Read the model definition and answer for the solid it produces. Units are mm, in the model's axes. A direction names the side the tool comes from. Give positions to 0.01 mm unless a question says otherwise; leave off trailing zeros. Loops run counter-clockwise (first coordinate to the right, second up) from the corner with the lowest first, then second, coordinate; pieces in that order, holes last. Notation, with made-up numbers: (21.25, 66) -> (39.25, 66) arc R13 cw to (39.25, 74) -> close; hole circle Ø7 at (57.25, 50.25). An arc over 180 degrees is marked (long way). Write each question's results on one line, items separated by ' | '. Start each with the question number.
Item 1: Find the intervals of material crossed by line 1 (Z direction, x = 6.5, y = 6); line 2 (Z direction, x = 51, y = 3.5); line 3 (Z direction, x = -26, y = 2.75), in increasing order.
Item 2: Which of the six approach directions +Z, -Z, +X, -X, +Y, -Y give full straight-line access (tool end or side, diameter ignored) to faces 1 (the flat face through (35, 3, 36.341)), 2 (the flat face through (-38.148, 3, 41))?
Item 3: Section B-B on y = 2.25 is taken. Write down the section's boundary in (x, z) (1 decimal).
Item 4: Each of these flat-tipped pins is pushed along its axis until it touches: P1, Ø2, axis at x = -27, y = 2, coming from the -Z side; P2, Ø3, axis at x = 50.75, z = 79.44, coming from the -Y side. Where does it stop, or does it pass through?
Item 5: Section A-A on x = 46 is taken. Write down the section's boundary in (y, z).
Item 6: Determine the mould class of faces 3 (the cylindrical face through (4.254, 3.131, 41.423)), 4 (the cylindrical face through (-34.329, 3.131, -5.834)), 5 (the flat face through (1, 6.35, 41)) for opening direction Z: +Z half, -Z half, draft (parallel to the pull), parting line (faces both ways), or undercut.
```python
from build123d import *

# Parameters (mm, degrees)
SKETCH1_R           = 1.5875
BOSS_EXTRUDE1_DEPTH = 6.35


with BuildPart() as part:
    # Sketch1 → Boss-Extrude1 (new body)
    with BuildSketch(Plane(origin=(0, 0, 0), x_dir=(1, 0, 0), z_dir=(0, 1, 0))):
        with BuildLine():
            Line((63.451864614, -36.34068615), (63.451864614, -3.24448615))
            ThreePointArc((63.451864614, -3.24448615), (59.732120735, 5.735769971), (50.751864614, 9.45551385))
            Line((50.751864614, 9.45551385), (-25.448135386, 9.45551385))
            ThreePointArc((-25.448135386, 9.45551385), (-34.428391507, 5.735769971), (-38.148135386, -3.24448615))
            Line((-38.148135386, -3.24448615), (-38.148135386, -79.44448615))
            ThreePointArc((-38.148135386, -79.44448615), (-34.428391507, -88.424742271), (-25.448135386, -92.14448615))
            Line((-25.448135386, -92.14448615), (50.751864614, -92.14448615))
            ThreePointArc((50.751864614, -92.14448615), (59.732120735, -88.424742271), (63.451864614, -79.44448615))
            Line((63.451864614, -79.44448615), (63.451864614, -46.34828615))
            Line((63.451864614, -46.34828615), (18.246283087, -46.34828615))
            Line((18.246283087, -46.34828615), (6.358123925, -46.34828615))
            ThreePointArc((6.358123925, -46.34828615), (4.253221481, -41.34448615), (6.358123925, -36.34068615))
            Line((6.358123925, -36.34068615), (18.246283087, -36.34068615))
            Line((18.246283087, -36.34068615), (63.451864614, -36.34068615))
        make_face()
        with Locations(Location((-25.448135386, -79.44448615, 0), (0, 0, 270))):
            Circle(SKETCH1_R, mode=Mode.SUBTRACT)
        with Locations(Location((50.751864614, -79.44448615, 0), (0, 0, 270))):
            Circle(SKETCH1_R, mode=Mode.SUBTRACT)
        with Locations(Location((50.751864614, -3.24448615, 0), (0, 0, 270))):
            Circle(SKETCH1_R, mode=Mode.SUBTRACT)
        with Locations(Location((-25.448135386, -3.24448615, 0), (0, 0, 270))):
            Circle(SKETCH1_R, mode=Mode.SUBTRACT)
    extrude(amount=BOSS_EXTRUDE1_DEPTH)


solid = part.part
```
Findings:
1) line 1: -9.46 to 36.34, 46.35 to 92.14 | line 2: -9.45 to 1.68, 4.81 to 36.34, 46.35 to 77.88, 81.01 to 92.14 | line 3: -9.44 to 1.76, 4.73 to 77.96, 80.93 to 92.13
2) face 1: +X, +Y, -Y | face 2: +Z, -Z, -X, +Y, -Y
3) outline: (-38.1, 3.2) arc R12.7 ccw to (-25.4, -9.5) -> (50.8, -9.5) arc R12.7 ccw to (63.5, 3.2) -> (63.5, 36.3) -> (6.4, 36.3) arc R7 cw to (6.4, 46.3) -> (63.5, 46.3) -> (63.5, 79.4) arc R12.7 ccw to (50.8, 92.1) -> (-25.4, 92.1) arc R12.7 ccw to (-38.1, 79.4) -> close; hole circle Ø3.2 at (-25.4, 3.2); hole circle Ø3.2 at (-25.4, 79.4); hole circle Ø3.2 at (50.8, 3.2); hole circle Ø3.2 at (50.8, 79.4)
4) P1: z = -9.44 | P2: through
5) outline: (0, -9.46) -> (6.35, -9.46) -> (6.35, 36.34) -> (0, 36.34) -> close; (0, 46.35) -> (6.35, 46.35) -> (6.35, 92.14) -> (0, 92.14) -> close
6) face 3: undercut | face 4: -Z half | face 5: draft
